The listing builds one solid part. Answer for the finished solid, in the listing's coordinates (mm). Face numbers are marked on the shaded views. Round coordinates to 2 decimals unless told otherwise and drop trailing zeros. Write each loop counter-clockwise with the first axis right and the second up, starting at its lowest first coordinate (ties: lowest second). Pieces come first, ordered by that corner, then holes.
(1) A cutting plane is placed at D-D, the plane y = -7.75. Give the vertices of the cut face in (x, z), and give its area (3 significant figures).
(2) A cutting plane is placed at A-A, the plane y = 0. Give the vertices of the cut face in (x, z), and give its area (3 significant figures).
(3) Each of these flat-tipped pins is pushed along its axis until it touches: pin 1 Ø12 at (x, z) = (6.5, 34) entering from -Y; pin 2 Ø10 at (y, z) = (-1, 37) entering from +X; pin 3 Ø1 at (x, z) = (3, 46.5) entering from +Y; pin 4 Ø5 at (x, y) = (-4, 4) entering from -Z. Where does it stop, or does it pass through?
(4) Find the intervals of material crossed by probe 1 along X at (y, z) = (0, 16); probe 2 along Z at (x, y) = (-0.5, -7.25), in increasing order.
(5) A cutting plane is placed at B-B, the plane x = 0. Give the vertices of the cut face in (y, z).
(6) A cutting plane is placed at C-C, the plane z = 16.5. Give the vertices of the cut face in (x, y), and give its area (3 significant figures).
(7) The mould has two halves that part along X. Classify the marked faces 1 and 2: +X half, -X half, draft (parallel to the pull), parting line (faces both ways), or undercut.
from build123d import *

# Parameters (mm, degrees)
SKETCH_R          = 10
PAD_DEPTH         = 60
CYLINDER_R        = 7
CYLINDER_DEPTH    = 70
CYLINDER001_R     = 22.5
CYLINDER001_DEPTH = 25


with BuildPart() as part:
    # Sketch → Pad (new body)
    with BuildSketch(Plane.XY):
        Circle(SKETCH_R)
    extrude(amount=PAD_DEPTH)

    # Cylinder → Cylinder (cut)
    with BuildSketch(Plane.XY.offset(-6)):
        Circle(CYLINDER_R)
    extrude(amount=CYLINDER_DEPTH, mode=Mode.SUBTRACT)

    # Cylinder001 → Cylinder001 (cut)
    with BuildSketch(Plane(origin=(0, 12, -19), x_dir=(1, 0, 0), z_dir=(0, -1, 0))):
        Circle(CYLINDER001_R)
    extrude(amount=CYLINDER001_DEPTH, mode=Mode.SUBTRACT)


solid = part.part
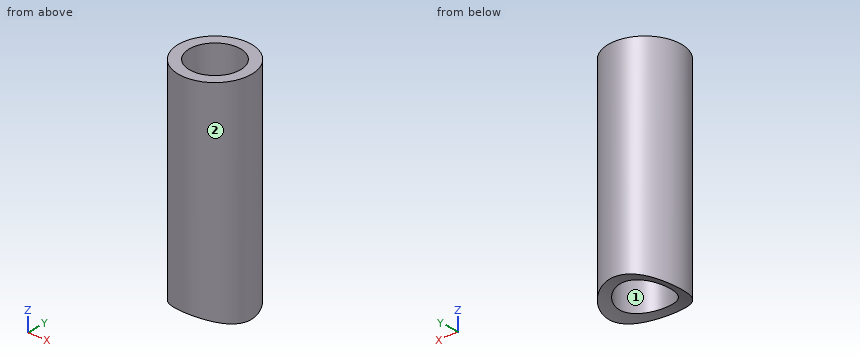
Solutions:
1. outline: (-6.32, 2.59) arc R22.5 cw to (6.32, 2.59) - (6.32, 60) - (-6.32, 60) - close
1. area: 718 mm2
2. outline: (-10, 1.16) arc R22.5 cw to (-7, 2.38) - (-7, 60) - (-10, 60) - close; (7, 2.38) arc R22.5 cw to (10, 1.16) - (10, 60) - (7, 60) - close
2. area: 349 mm2
3. pin 1: stops at y = -9.99
3. pin 2: stops at x = 10
3. pin 3: stops at y = 9.68
3. pin 4: stops at z = 2.54
4. probe 1: x = -10 to -7, 7 to 10
4. probe 2: z = 3.49 to 60
5. outline: (-10, 3.5) - (-7, 3.5) - (-7, 60) - (-10, 60) - close; (7, 3.5) - (10, 3.5) - (10, 60) - (7, 60) - close
6. outline: circle Ø20 at (0, 0); hole circle Ø14 at (0, 0)
6. area: 160 mm2
7. face 1: undercut
7. face 2: parting line
